from build123d import *

# Parameters (mm, degrees)
SKETCH_1_R           = 7
EXTRUDE_1_DEPTH      = 34
EXTRUDE_2_DEPTH      = 2
EXTRUDE_2_DEPTH_BACK = 3
SKETCH_2_R           = 12
EXTRUDE_4_DEPTH      = 3


with BuildPart() as part:
    # 草图1 → 凸台-拉伸1 (new body)
    with BuildSketch(Plane.XY):
        with Locations((-86.606649797, -63.783530386)):
            Circle(SKETCH_1_R)
    extrude(amount=EXTRUDE_1_DEPTH)

    # 草图2 → 凸台-拉伸2 (add, two sides: drawn at the far end of the back side and taken through both)
    with BuildSketch(Plane.XY.offset(34).offset(-EXTRUDE_2_DEPTH_BACK)):
        with Locations((-86.606649797, -63.783530386)):
            Circle(SKETCH_2_R)
    extrude(amount=EXTRUDE_2_DEPTH + EXTRUDE_2_DEPTH_BACK)

    # 草图3 → 凸台-拉伸4 (add)
    with BuildSketch(Plane.XY.offset(36)):
        Polygon((-99.453609906, -46.708587879), (-56.43686088, -55.3563008), (-64.649842886, -96.21054618), (-107.666591911, -87.562833258), align=None)
    extrude(amount=EXTRUDE_4_DEPTH)


solid = part.part
Work out the finished part from the listing and answer in its coordinate system (mm). A direction names the side the tool comes from. Give positions to 0.01 mm unless a question says otherwise; leave off trailing zeros. Loops run counter-clockwise (first coordinate to the right, second up) from the corner with the lowest first, then second, coordinate; pieces in that order, holes last. Notation, with made-up numbers: (-39.75, 79) - (-13.75, 79) arc R16 cw to (-13.75, 94) - close; hole circle Ø8 at (67.5, 29). An arc over 180 degrees is marked (long way). Answer in a Markdown table with one row per item.
(1) Consider L1, parallel to Z at x = -79.5, y = -86; L2, parallel to X at y = -63.5, z = 12.5; L3, parallel to X at y = -67.5, z = 9. Determine where each line is inside the solid, lowest interval first. Write a range as [from, to].
Results list:
| item | result |
|---|---|
| L1 | z = [36, 39] |
| L2 | x = [-93.6, -79.61] |
| L3 | x = [-92.54, -80.67] |
(2) Section A-A (x = -82) is taken. Give the vertices of the cut face in (y, z), and give its area (3 significant figures).
Results list:
| item | result |
|---|---|
| outline | (-92.72, 36) - (-74.86, 36) - (-74.86, 31) - (-69.05, 31) - (-69.05, 0) - (-58.51, 0) - (-58.51, 31) - (-52.7, 31) - (-52.7, 36) - (-50.22, 36) - (-50.22, 39) - (-92.72, 39) - close |
| area | 565 mm² |
(3) A tool of negligible diameter and unlimited length cuts with its end or side. For faces 1 (the face through (-103.618, -67.422, 37.479)), 2 (the face through (-87.518, -56.843, 15.283)), from which of +Z, -Z, +X, -X, +Y, -Y can it reach the whole face along a straight path? Write none if from no direction.
Results list:
| item | result |
|---|---|
| face 1 | +Z, -Z, -X, +Y |
| face 2 | -Z |
(4) Section B-B (y = -66) is taken. Give the vertices of the cut face in (x, z), and give its area (3 significant figures).
Results list:
| item | result |
|---|---|
| outline | (-103.33, 36) - (-98.4, 36) - (-98.4, 31) - (-93.25, 31) - (-93.25, 0) - (-79.97, 0) - (-79.97, 31) - (-74.81, 31) - (-74.81, 36) - (-58.58, 36) - (-58.58, 39) - (-103.33, 39) - close |
| area | 664 mm² |
(5) Section D-D (y = -53) is taken. Give the vertices of the cut face in (x, z), and give its area (3 significant figures).
Results list:
| item | result |
|---|---|
| outline | (-100.72, 36) - (-91.87, 36) - (-91.87, 31) - (-81.34, 31) - (-81.34, 36) - (-68.16, 36) - (-68.16, 39) - (-100.72, 39) - close |
| area | 150 mm² |
(6) Flat-ended cylindrical pins translate along their axes: pin 1 Ø10 at (y, z) = (-72.5, 8) entering from -X; pin 2 Ø6 at (x, z) = (-78.5, 17.5) entering from -Y; pin 3 Ø3 at (x, y) = (-63, -57) entering from -Z. Find the tip coordinate at first contact, or state that the pin passes through.
Results list:
| item | result |
|---|---|
| pin 1 | stops at x = -92.54 |
| pin 2 | stops at y = -68.57 |
| pin 3 | stops at z = 36 |
(7) Section C-C (z = 13.5) is taken. Give the vertices of the cut face in (x, y), and give its area (3 significant figures).
Results list:
| item | result |
|---|---|
| outline | circle Ø14 at (-86.61, -63.78) |
| area | 154 mm² |
